Design review of the part shown in the three views and the two pictorial views. Dimensions are in mm from the part's minimum x, y and z. Coordinates: 2 decimals unless noted, no trailing zeros. Write each loop counter-clockwise with the first axis right and the second up, starting at its lowest first coordinate (ties: lowest second). Pieces come first, ordered by that corner, then holes. Notation, with made-up numbers: M 22,77 L 65,77 A4 ccw 65,81 Z; hole C 77.5,-0.75 d3. An arc over 180 degrees is marked long. One line per question, with ' | ' between items.
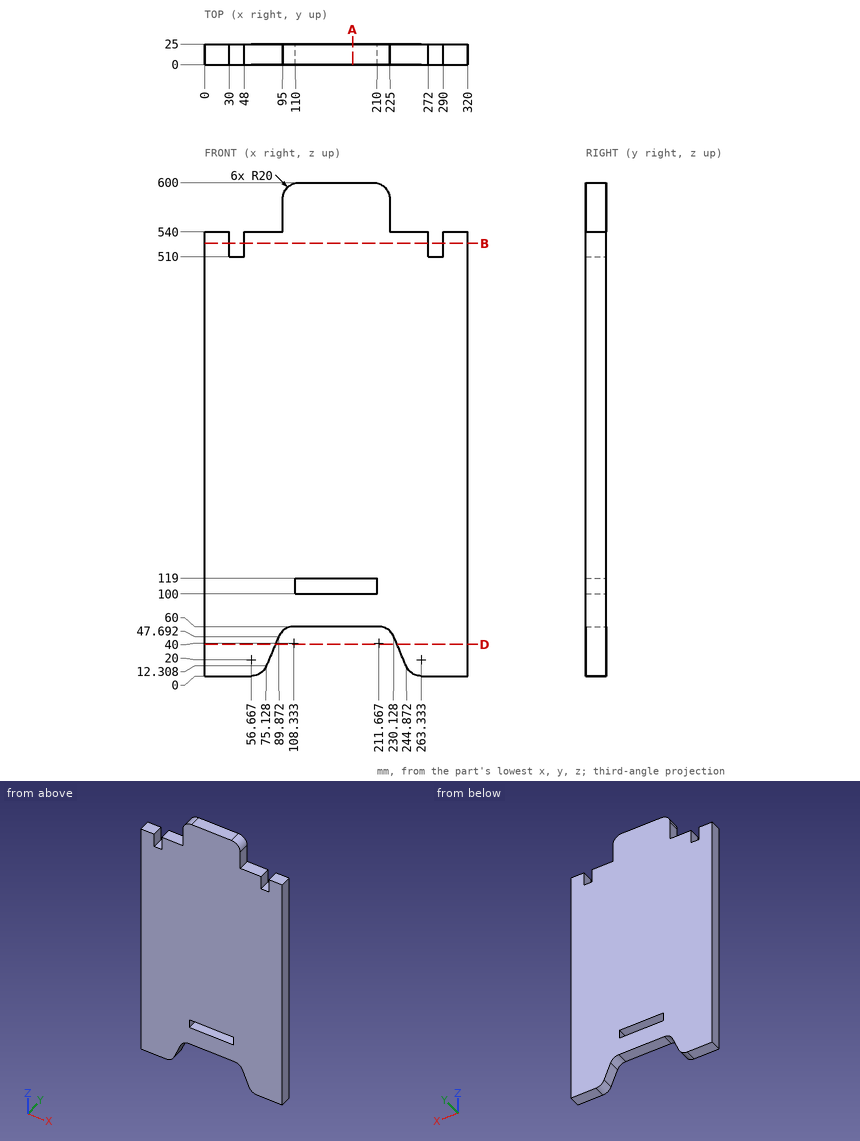
1. Clearance check with flat-ended pins moving along their axes: P1, Ø12.5, axis at y = 6.5, z = 560.5, coming from the -X side; P2, Ø8, axis at x = 62, y = 18, coming from the +Z side; P3, Ø5.5, axis at x = 35.5, y = 17, coming from the +Z side. State where each tip first meets the part, or that it passes through.
Computed values:
P1: stops at x = 95 | P2: stops at z = 540 | P3: stops at z = 510
2. For line 1 along X through (y, z) = (2, 511.5); line 2 along X through (y, z) = (14.5, 105); line 3 along Z through (x, y) = (189, 14), list the stretches that pass through material, from the lowest coordinate up.
Computed values:
line 1: x = 0 to 30, 48 to 272, 290 to 320 | line 2: x = 0 to 110, 210 to 320 | line 3: z = 60 to 100, 119 to 600
3. Take a section at D-D on z = 38.5. State the section outline as (x, y) points, plus the area to 3 significant figures.
Computed values:
outline: M 0,0 L 86.04,0 L 86.04,25 L 0,25 Z; M 233.96,0 L 320,0 L 320,25 L 233.96,25 Z | area: 4,300 mm2
4. Take a section at B-B on z = 526. State the section outline as (x, y) points, plus the area to 3 significant figures.
Computed values:
outline: M 0,0 L 30,0 L 30,25 L 0,25 Z; M 48,0 L 272,0 L 272,25 L 48,25 Z; M 290,0 L 320,0 L 320,25 L 290,25 Z | area: 7,100 mm2
5. Take a section at A-A on x = 180. State the section outline as (y, z) points.
Computed values:
outline: M 0,60 L 25,60 L 25,100 L 0,100 Z; M 0,119 L 25,119 L 25,600 L 0,600 Z
